Drawing for the job (mm, zero at the part's lowest x, y, z). A direction names the side the tool comes from. Round coordinates to 2 decimals unless told otherwise and drop trailing zeros. Order: outer loops, then holes, each group sorted by start corner. A loop starts at its lowest first (then second) coordinate and runs counter-clockwise, first axis right, second up. Notation, with made-up numbers: (3, -28.5) -> (30, -28.5) arc R24 cw to (30, -17.5) -> close; hole circle Ø7 at (-29.5, -12.5). An arc over 180 degrees is marked (long way). Use CSV: the item, a comma, the result in double quotes.
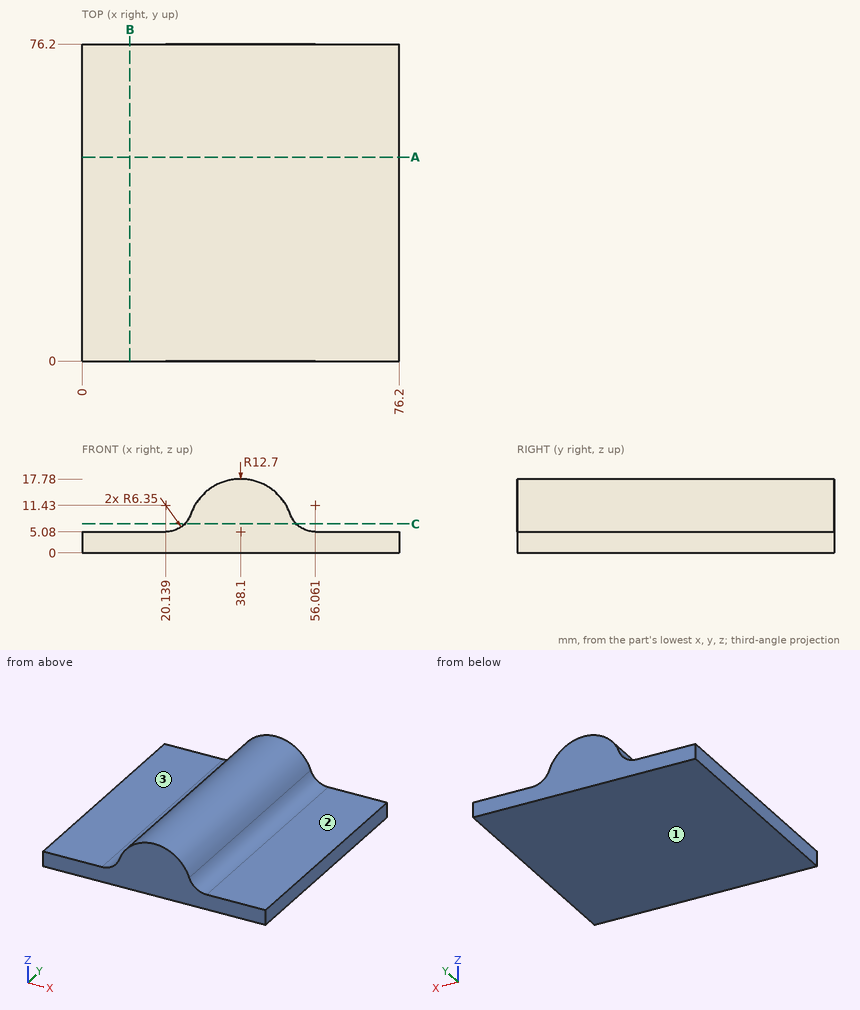
Q1. Cut at C-C (z = 7). Give the cut face in (x, y).
From the geometry:
outline,"(24.69, 0) -> (51.51, 0) -> (51.51, 76.2) -> (24.69, 76.2) -> close"
Q2. Pin check, flat tips, straight feed: pin 1 (5 mm diameter, centred on x = 58.5, z = 6, fed in from -Y); pin 2 (22 mm diameter, centred on x = 66, y = 54.5, fed in from +Z); pin 3 (6 mm diameter, centred on x = 14.5, y = 44, fed in from +Z); pin 4 (4 mm diameter, centred on x = 21, y = 27, fed in from +Z). Stop position of each tip, or through.
From the geometry:
pin 1,"stops at y = 0"
pin 2,"stops at z = 5.17"
pin 3,"stops at z = 5.08"
pin 4,"stops at z = 5.76"
Q3. Cut at B-B (x = 11.5). Give the cut face in (y, z).
From the geometry:
outline,"(0, 0) -> (76.2, 0) -> (76.2, 5.08) -> (0, 5.08) -> close"
Q4. Which spindle directions (+Z, -Z, +X, -X, +Y, -Y) get a long thin tool onto all of the face, cutting with end or side? Do the marked faces 1, 2 and 3. Say none if no direction does.
From the geometry:
face 1,"-Z, +X, -X, +Y, -Y"
face 2,"+Z, +X, +Y, -Y"
face 3,"+Z, -X, +Y, -Y"
Q5. Cut at A-A (y = 49). Give the cut face in (x, z), plus the area to 3 significant figures.
From the geometry:
outline,"(0, 0) -> (76.2, 0) -> (76.2, 5.08) -> (56.06, 5.08) arc R6.35 cw to (50.07, 9.31) arc R12.7 ccw to (26.13, 9.31) arc R6.35 cw to (20.14, 5.08) -> (0, 5.08) -> close"
area,"650 mm²"
Q6. Probe line 1 along Z through (x, y) = (8, 36.5); line 2 along Z through (x, y) = (49, 50.5) (1 decimal); line 3 along X through (y, z) = (24, 11) (1 decimal). List the from-to ranges inside material, lowest first.
From the geometry:
line 1,"z = 0 to 5.08"
line 2,"z = 0 to 11.6"
line 3,"x = 26.9 to 49.3"
